Build history of the part. All positions in model axes, mm. Face numbers are marked on the shaded views. A direction names the side the tool comes from. Round coordinates to 2 decimals unless told otherwise and drop trailing zeros. Order: outer loops, then holes, each group sorted by start corner. A loop starts at its lowest first (then second) coordinate and runs counter-clockwise, first axis right, second up. Notation, with made-up numbers: M 19,61.25 L 77,61.25 A13 cw 77,73.25 Z; hole C 65,73 d1. An arc over 180 degrees is marked long. One line per item, written item: value. Start each with the question number.
Item 1: Band-saw the part on D-D, the plane y = -43. Write the cut outline in (x, z), then the cut area to 3 significant figures.
Item 2: Pin check, flat tips, straight feed: pin 1 (2.5 mm diameter, centred on x = -2.5, z = 5.5, fed in from +Y); pin 2 (2.5 mm diameter, centred on y = -32.5, z = 5, fed in from +X); pin 3 (6 mm diameter, centred on x = 7.5, y = -31, fed in from +Z); pin 4 (4 mm diameter, centred on y = -33, z = 5.5, fed in from -X). Stop position of each tip, or through.
Item 3: Band-saw the part on C-C, the plane z = 6.75. Write the cut outline in (x, y).
Item 4: Probe L1, parallel to Y at x = -38, z = 5.5; L2, parallel to X at y = -30.5, z = 0.5. List the from-to ranges inside material, lowest first.
Item 5: Band-saw the part on B-B, the plane y = -36. Write the cut outline in (x, z).
Item 6: Two-plate mould, pull along X, no slides. Class the marked faces 3, 4 and 5: +X half, -X half, draft (parallel to the pull), parting line (faces both ways), or undercut.
Item 7: Tool access for the marked faces 1 and 2: list every direction of +Z, -Z, +X, -X, +Y, -Y with a clear straight run to the whole face (end or side of a thin tool).
Item 8: Band-saw the part on A-A, the plane z = 4. Write the cut outline in (x, y), then the cut area to 3 significant figures.
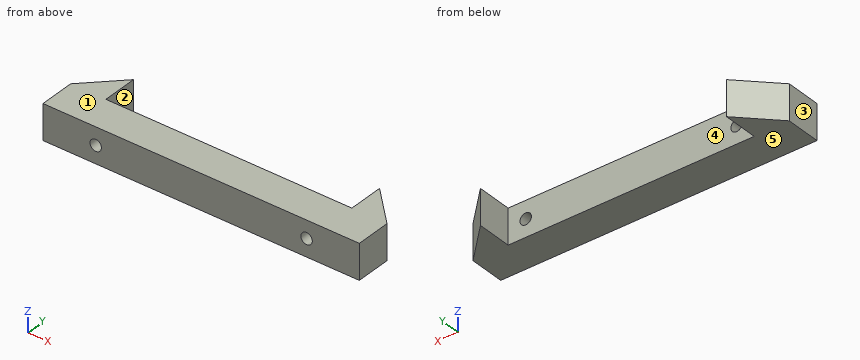
```python
from build123d import *

# Parameters (mm, degrees)
BOSS_EXTRUDE1_DEPTH = 8
CUT_EXTRUDE1_REACH  = 53.887
SKETCH2_R           = 1.3


with BuildPart() as part:
    # Sketch1 → Boss-Extrude1 (new body)
    with BuildSketch(Plane(origin=(0, 0, 0), x_dir=(0, 1, 0), z_dir=(0, 0, 1))):
        Polygon((-44.64033264, 50.63902284), (-44.64033264, -21.36097716), (-36.64033264, -21.36097716), (-28.64033264, -13.36097716), (-36.64033264, -13.36097716), (-36.64033264, 42.63902284), (-28.64033264, 42.63902284), (-36.64033264, 50.63902284), align=None)
    extrude(amount=BOSS_EXTRUDE1_DEPTH)

    # Sketch2 → Cut-Extrude1 (cut, up to next)
    with BuildSketch(Plane(origin=(0, -36.64033264, 0), x_dir=(-1, 0, 0), z_dir=(0, 1, 0)), mode=Mode.PRIVATE) as cut_extrude1_sk1:
        with Locations(Location((-9.36097716, 4, 0), (0, 0, 90))):
            Circle(SKETCH2_R)
    cut_extrude1_tool1 = extrude(cut_extrude1_sk1.sketch, amount=-CUT_EXTRUDE1_REACH, mode=Mode.PRIVATE) & part.part
    # Sketch2 → Cut-Extrude1 (cut, up to next)
    with BuildSketch(Plane(origin=(0, -36.64033264, 0), x_dir=(-1, 0, 0), z_dir=(0, 1, 0)), mode=Mode.PRIVATE) as cut_extrude1_sk2:
        with Locations((38.63902284, 4)):
            Circle(SKETCH2_R)
    cut_extrude1_tool2 = extrude(cut_extrude1_sk2.sketch, amount=-CUT_EXTRUDE1_REACH, mode=Mode.PRIVATE) & part.part
    add(cut_extrude1_tool1.solids().sort_by_distance((9.360977, -36.640333, 4))[0], mode=Mode.SUBTRACT)
    add(cut_extrude1_tool2.solids().sort_by_distance((-38.639023, -36.640333, 4))[0], mode=Mode.SUBTRACT)


solid = part.part
```
Output:
1. outline: M -50.64,0 L 21.36,0 L 21.36,8 L -50.64,8 Z; hole C -38.64,4 d2.6; hole C 9.36,4 d2.6
1. area: 565 mm²
2. pin 1: stops at y = -36.64
2. pin 2: stops at x = 18.47
2. pin 3: passes through
2. pin 4: stops at x = -49
3. outline: M -50.64,-44.64 L 21.36,-44.64 L 21.36,-36.64 L 13.36,-28.64 L 13.36,-36.64 L -42.64,-36.64 L -42.64,-28.64 L -50.64,-36.64 Z
4. L1: y = -44.64 to -36.64
4. L2: x = -44.5 to -42.64, 13.36 to 15.22
5. outline: M -50,0 L -42.64,0 L -42.64,8 L -50,8 Z; M 13.36,0 L 20.72,0 L 20.72,8 L 13.36,8 Z
6. face 3: -X half
6. face 4: undercut
6. face 5: draft
7. face 1: +Z, +X, -X, +Y, -Y
7. face 2: +Z, -Z, +Y
8. outline: M -50.64,-44.64 L -39.94,-44.64 L -39.94,-36.64 L -42.64,-36.64 L -42.64,-28.64 L -50.64,-36.64 Z; M -37.34,-44.64 L 8.06,-44.64 L 8.06,-36.64 L -37.34,-36.64 Z; M 10.66,-44.64 L 21.36,-44.64 L 21.36,-36.64 L 13.36,-28.64 L 13.36,-36.64 L 10.66,-36.64 Z
8. area: 598 mm²
